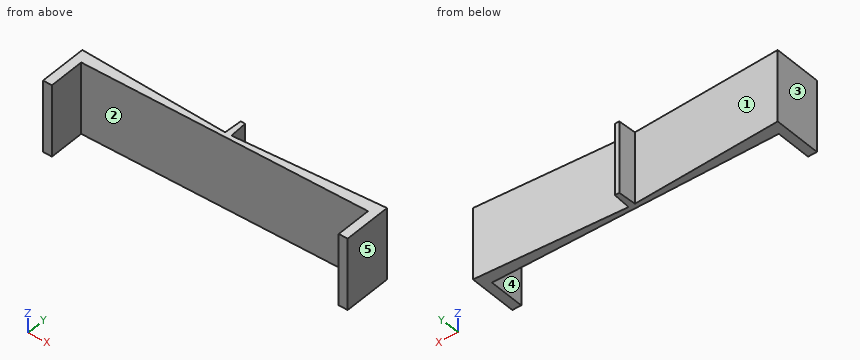
```python
from build123d import *

# Parameters (mm, degrees)
SKETCH3_W           = 53.975
SKETCH3_H           = 1.5875
SKETCH3_W_2         = 3.175
SKETCH3_H_2         = 12.7
BOSS_EXTRUDE2_DEPTH = 25.4


with BuildPart() as part:
    # Sketch3 → Boss-Extrude2 (new body)
    with BuildSketch(Plane.XY):
        with Locations((26.9875, 0.79375)):
            Rectangle(SKETCH3_W, SKETCH3_H)
        with Locations((52.3875, -6.35)):
            Rectangle(SKETCH3_W_2, SKETCH3_H_2)
        Polygon((53.975, 4.357170459), (1.126539398, 1.5875), (53.975, 1.5875), align=None)
        Polygon((0, 7.9375), (0, 1.5875), (1.126539398, 1.5875), (0.79375, 7.9375), align=None)
    boss_extrude2 = extrude(amount=BOSS_EXTRUDE2_DEPTH)

    # Mirror1: Boss-Extrude2 across plane
    add(boss_extrude2.mirror(Plane(origin=(0, 0, 0), x_dir=(0, 0, 1), z_dir=(1, 0, 0))))


solid = part.part
```
Work out the finished part from the listing and answer in its coordinate system (mm). Face numbers are marked on the shaded views. A direction names the side the tool comes from. Give positions to 0.01 mm unless a question says otherwise; leave off trailing zeros. Loops run counter-clockwise (first coordinate to the right, second up) from the corner with the lowest first, then second, coordinate; pieces in that order, holes last. Notation, with made-up numbers: (78.5, 87) -> (87.5, 87) arc R14 ccw to (87.5, 112) -> close; hole circle Ø7 at (-1, 31.5). An arc over 180 degrees is marked (long way). One line per question, with ' | ' between items. Start each with the question number.
1) Section C-C, the plane x = 37 is taken. Determine the outline of the cut face in (y, z), then the cut area to 3 significant figures.
2) For the marked faces 1 and 2, determine the directions among +Z, -Z, +X, -X, +Y, -Y from which every point of the face is accessible in a straight line to the end or side of a thin tool.
3) Determine the mould class of the marked faces 3, 4 and 5 for opening direction X: +X half, -X half, draft (parallel to the pull), parting line (faces both ways), or undercut.
4) Each of these flat-tipped pins is pushed along its axis until it touches: pin 1 (12 mm diameter, centred on x = -12.5, z = 17.5, fed in from +Y); pin 2 (10 mm diameter, centred on x = 16.5, z = 12, fed in from -Y); pin 3 (6 mm diameter, centred on x = 9, y = -2.5, fed in from +Z). Where does it stop, or does it pass through?
5) Section B-B, the plane z = 8.25 is taken. Determine the outline of the cut face in (x, y) (1 decimal).
6) Section A-A, the plane y = -9.5 is taken. Determine the outline of the cut face in (x, z) (3 decimals).
7) Straight lines are drawn through the part: L1, parallel to X at y = -2, z = 17.5 (3 decimals); L2, parallel to Y at x = -41, z = 14.75; L3, parallel to Y at x = 31, z = 22.75. For each, find the intervals that lie inside material, in ascending order.
8) Section D-D, the plane x = -24 is taken. Determine the outline of the cut face in (y, z).
Resolved:
1) outline: (0, 0) -> (3.47, 0) -> (3.47, 25.4) -> (0, 25.4) -> close | area: 88.1 mm2
2) face 1: +Z, -Z, +Y | face 2: +Z, -Z, -Y
3) face 3: -X half | face 4: undercut | face 5: +X half
4) pin 1: y = 2.5 | pin 2: y = 0 | pin 3: z = 25.4
5) outline: (-54, -12.7) -> (-50.8, -12.7) -> (-50.8, 0) -> (50.8, 0) -> (50.8, -12.7) -> (54, -12.7) -> (54, 4.4) -> (1.1, 1.6) -> (0.8, 7.9) -> (-0.8, 7.9) -> (-1.1, 1.6) -> (-54, 4.4) -> close
6) outline: (-53.975, 0) -> (-50.8, 0) -> (-50.8, 25.4) -> (-53.975, 25.4) -> close; (50.8, 0) -> (53.975, 0) -> (53.975, 25.4) -> (50.8, 25.4) -> close
7) L1: -53.975 to -50.8, 50.8 to 53.975 | L2: 0 to 3.68 | L3: 0 to 3.15
8) outline: (0, 0) -> (2.79, 0) -> (2.79, 25.4) -> (0, 25.4) -> close
